Verification items for the finished model (mm, model axes). Face numbers are marked on the shaded views. A direction names the side the tool comes from. Give positions to 0.01 mm unless a question says otherwise; leave off trailing zeros. Loops run counter-clockwise (first coordinate to the right, second up) from the corner with the lowest first, then second, coordinate; pieces in that order, holes last. Notation, with made-up numbers: (43, 81.5) - (47, 81.5) arc R28 ccw to (47, 105.5) - close; hole circle Ø6 at (86.5, 54). An arc over 180 degrees is marked (long way). Answer in a Markdown table with one row per item.
```python
from build123d import *

# Parameters (mm, degrees)
BOSS_EXTRUDE1_DEPTH = 1.2
SKETCH2_W           = 4.5
SKETCH2_H           = 1
BOSS_EXTRUDE2_DEPTH = 2.66
FILLET1_R           = 1
SKETCH3_R           = 1
CUT_EXTRUDE1_DEPTH  = 0.1
SKETCH4_R           = 1
BOSS_EXTRUDE3_DEPTH = 5
FILLET2_R           = 0.2


with BuildPart() as part:
    # Sketch1 → Boss-Extrude1 (new body)
    with BuildSketch(Plane.XY):
        with BuildLine():
            Line((-2.25, 0), (-2.25, -2.25))
            Line((-2.25, -2.25), (2.25, -2.25))
            Line((2.25, -2.25), (2.25, 0))
            ThreePointArc((2.25, 0), (0, 2.25), (-2.25, 0))
        make_face()
    extrude(amount=BOSS_EXTRUDE1_DEPTH)

    # Sketch2 → Boss-Extrude2 (add)
    with BuildSketch(Plane.XY):
        with Locations((0, -2.75)):
            Rectangle(SKETCH2_W, SKETCH2_H)
    extrude(amount=BOSS_EXTRUDE2_DEPTH)

    # Fillet1
    fillet1_edges = [part.edges().sort_by_distance(p)[0] for p in [
        (0, -2.25, 2.66),
    ]]
    fillet(fillet1_edges, radius=FILLET1_R - 0.0001)  # a hair under: the kernel refuses the full size

    # Sketch3 → Cut-Extrude1 (cut)
    with BuildSketch(Plane.XY.offset(1.2)):
        Circle(SKETCH3_R)
    extrude(amount=-CUT_EXTRUDE1_DEPTH, mode=Mode.SUBTRACT)

    # Sketch4 → Boss-Extrude3 (add)
    with BuildSketch(Plane(origin=(0, 0, 0), x_dir=(-1, 0, 0), z_dir=(0, 0, -1))):
        with Locations(Location((0, 0, 0), (0, 0, 180))):
            Circle(SKETCH4_R)
    extrude(amount=BOSS_EXTRUDE3_DEPTH)

    # Fillet2
    fillet2_edges = [part.edges().sort_by_distance(p)[0] for p in [
        (-1, 0, -5),
    ]]
    fillet(fillet2_edges, radius=FILLET2_R)


solid = part.part
```
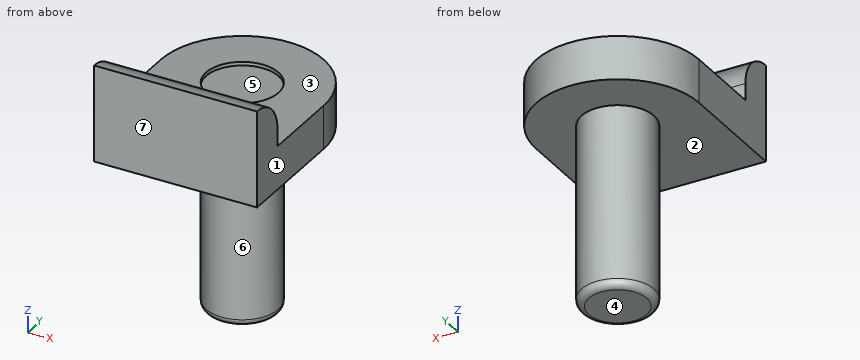
Q1. Thickness scan on line 1 (Y direction, x = 0, z = 1.15); line 2 (Y direction, x = 0, z = 1.25); line 3 (X direction, y = 0.05, z = -2.5). Record the ranges inside material, lowest first.
Completed:
| item | result |
|---|---|
| line 1 | -3.25 to -1, 1 to 2.25 |
| line 2 | -3.25 to -2.25 |
| line 3 | -1 to 1 |
Q2. Draft check along Y on the marked faces 4, 5, 6 and 7. Enter one of: +Y half, -Y half, draft (parallel to the pull), parting line (faces both ways), or undercut.
Completed:
| item | result |
|---|---|
| face 4 | draft |
| face 5 | undercut |
| face 6 | parting line |
| face 7 | -Y half |
Q3. Tool access check on the marked faces 1, 2 and 3. Record the directions out of +Z, -Z, +X, -X, +Y, -Y that give a thin tool (end or side, any length) a straight path to the whole face; none if there is none.
Completed:
| item | result |
|---|---|
| face 1 | +Z, -Z, +X, +Y, -Y |
| face 2 | -Z |
| face 3 | +Z, +X, -X, +Y |
Q4. Sectioned sample at C-C (y = -1.8). Record the cut outline in (x, z), and give its area (3 significant figures).
Completed:
| item | result |
|---|---|
| outline | (-2.25, 0) - (2.25, 0) - (2.25, 1.2) - (-2.25, 1.2) - close |
| area | 5.40 mm^2 |
Q5. Go/stop test with flat-tipped pins: P1, Ø1, axis at y = 1.5, z = 0, coming from the +X side; P2, Ø2, axis at x = 0.5, y = 0.5, coming from the +Z side. Record where each tip stops, or that it passes through.
Completed:
| item | result |
|---|---|
| P1 | x = 2.02 |
| P2 | z = 1.2 |
Q6. Sectioned sample at B-B (z = 0.75). Record the cut outline in (x, y), and give its area (3 significant figures).
Completed:
| item | result |
|---|---|
| outline | (-2.25, -3.25) - (2.25, -3.25) - (2.25, 0) arc R2.25 ccw to (-2.25, 0) - close |
| area | 22.6 mm^2 |
